```python
from build123d import *

# Parameters (mm, degrees)
F1_DEPTH = 25.4


with BuildPart() as f1:
    # F0 (on Top) → F1 (new body)
    with BuildSketch(Plane.XY):
        with BuildLine():
            Line((0, 609.6), (-1143, 609.6))
            Line((-1143, 609.6), (-1143, 0))
            Line((-1143, 0), (-1143, -457.2))
            Line((-1143, -457.2), (-635, -457.2))
            ThreePointArc((-635, -457.2), (-585.441073, -211.265558), (-444.5, -3.719295))
            Line((-444.5, -3.719295), (444.5, -3.719295))
            ThreePointArc((444.5, -3.719295), (585.441073, -211.265558), (635, -457.2))
            Line((635, -457.2), (1143, -457.2))
            Line((1143, -457.2), (1143, 0))
            Line((1143, 0), (1143, 609.6))
            Line((1143, 609.6), (0, 609.6))
        make_face()
        Polygon((-874.864551, 202.616595), (-546.491051, 66.153398), (-658.347487, -177.842677), (-742.352484, -361.085502), (-1065.394138, -212.991774), align=None, mode=Mode.SUBTRACT)
        Polygon((742.352484, -361.085502), (658.347487, -177.842677), (546.491051, 66.153398), (874.864551, 202.616595), (1065.394138, -212.991774), align=None, mode=Mode.SUBTRACT)
    extrude(amount=F1_DEPTH)


solid = f1.part
```
The model under review builds one solid part; all positions refer to its coordinate system, in mm. A direction names the side the tool comes from. Round coordinates to 2 decimals unless told otherwise and drop trailing zeros. Order: outer loops, then holes, each group sorted by start corner. A loop starts at its lowest first (then second) coordinate and runs counter-clockwise, first axis right, second up. Notation, with made-up numbers: (80, -17) - (88, -17) arc R32 cw to (88, 16) - close; hole circle Ø6 at (71.25, 42.25). An arc over 180 degrees is marked (long way). Answer in a Markdown table with one row per item.
(1) For line 1 (X direction, y = -15.5, z = 3); line 2 (X direction, y = -284, z = 8.25); line 3 (Y direction, x = 150, z = 13.25), list the stretches that pass through material, from the lowest coordinate up. Write a range as from..to.
Result set:
| item | result |
|---|---|
| line 1 | x = -1143..-974.86, -583.92..-456.21, 456.21..583.92, 974.86..1143 |
| line 2 | x = -1143..-910.5, -707.01..-610.92, 610.92..707.01, 910.5..1143 |
| line 3 | y = -3.72..609.6 |
(2) Take a section at D-D on x = -329. Write out the cut boundary in (y, z), plus the area to 3 significant figures.
Result set:
| item | result |
|---|---|
| outline | (-3.72, 0) - (609.6, 0) - (609.6, 25.4) - (-3.72, 25.4) - close |
| area | 15,600 mm2 |
(3) Take a section at C-C on y = -255.5. Write out the cut boundary in (x, z).
Result set:
| item | result |
|---|---|
| outline | (-1143, 0) - (-972.67, 0) - (-972.67, 25.4) - (-1143, 25.4) - close; (-693.95, 0) - (-602.11, 0) - (-602.11, 25.4) - (-693.95, 25.4) - close; (602.11, 0) - (693.95, 0) - (693.95, 25.4) - (602.11, 25.4) - close; (972.67, 0) - (1143, 0) - (1143, 25.4) - (972.67, 25.4) - close |
(4) Clearance check with a flat-ended pin moving along its axis: P1, Ø7.5, axis at x = 95, z = 16, coming from the -Y side. State where the tip first meets the part, or that it passes through.
Result set:
| item | result |
|---|---|
| P1 | stops at y = -3.72 |
(5) Take a section at A-A on x = 785. Write out the cut boundary in (y, z).
Result set:
| item | result |
|---|---|
| outline | (-457.2, 0) - (-341.53, 0) - (-341.53, 25.4) - (-457.2, 25.4) - close; (165.27, 0) - (609.6, 0) - (609.6, 25.4) - (165.27, 25.4) - close |
(6) Machinability: for faces 4 (the face through (-971.463, -8.097, 12.522)), 5 (the face through (-16, 202, 25.4)), 6 (the face through (584.063, -208.01, 12.522)), which of the approach directions +Z, -Z, +X, -X, +Y, -Y give a long, thin tool a straight path to every point of the face, cutting with its end or side? Answer none if there is none.
Result set:
| item | result |
|---|---|
| face 4 | +Z, -Z |
| face 5 | +Z, +X, -X, +Y, -Y |
| face 6 | +Z, -Z, -Y |
(7) Take a section at B-B on z = 19.25. Write out the cut boundary in (x, y).
Result set:
| item | result |
|---|---|
| outline | (-1143, -457.2) - (-635, -457.2) arc R635 cw to (-444.5, -3.72) - (444.5, -3.72) arc R635 cw to (635, -457.2) - (1143, -457.2) - (1143, 609.6) - (-1143, 609.6) - close; hole (-1065.39, -212.99) - (-742.35, -361.09) - (-546.49, 66.15) - (-874.86, 202.62) - close; hole (546.49, 66.15) - (742.35, -361.09) - (1065.39, -212.99) - (874.86, 202.62) - close |
(8) Mouldability with a two-part tool opening along Y and no side actions: class faces 1 (the face through (-586.8, -214.53, 12.52)), 2 (the face through (-16, 202, 0)), 3 (the face through (-712.98, 135.34, 12.52)) as released by +Y, released by -Y, zero draft, split by the parting line, or undercut.
Result set:
| item | result |
|---|---|
| face 1 | released by -Y |
| face 2 | zero draft |
| face 3 | undercut |
